Work out the finished part from the listing and answer in its coordinate system (mm). A direction names the side the tool comes from. Round coordinates to 2 decimals unless told otherwise and drop trailing zeros. Order: outer loops, then holes, each group sorted by start corner. A loop starts at its lowest first (then second) coordinate and runs counter-clockwise, first axis right, second up. Notation, with made-up numbers: M -6.5,-13.5 L 37.5,-13.5 A26 ccw 37.5,6.5 Z; hole C -16,-37 d3. An arc over 180 degrees is marked long. Return JSON: item names as keys, results as strings.
from build123d import *

# Parameters (mm, degrees)
SKETCH1_R           = 3.175
BOSS_EXTRUDE1_DEPTH = 88.9
CUT_EXTRUDE1_DEPTH  = 50.8
CUT_EXTRUDE2_START  = -6.5532
SKETCH3_R           = 3.175
SKETCH3_R_2         = 2.667
CUT_EXTRUDE2_DEPTH  = 0.7366


with BuildPart() as part:
    # Sketch1 → Boss-Extrude1 (new body)
    with BuildSketch(Plane(origin=(0, 0, 0), x_dir=(1, 0, 0), z_dir=(0, 1, 0))):
        Circle(SKETCH1_R)
    extrude(amount=BOSS_EXTRUDE1_DEPTH)

    # Sketch2 → Cut-Extrude1 (cut)
    with BuildSketch(Plane.XZ):
        Polygon((-2.5, 0), (-2.5, -1.957198253), (-3.175, -1.957198253), (-3.175, 1.957198253), (-2.5, 1.957198253), align=None)
    extrude(amount=-CUT_EXTRUDE1_DEPTH, mode=Mode.SUBTRACT)

    # Sketch3 → Cut-Extrude2 (cut)
    with BuildSketch(Plane(origin=(0, 88.9, 0), x_dir=(1, 0, 0), z_dir=(0, 1, 0)).offset(CUT_EXTRUDE2_START)):
        Circle(SKETCH3_R)
        Circle(SKETCH3_R_2, mode=Mode.SUBTRACT)
    extrude(amount=-CUT_EXTRUDE2_DEPTH, mode=Mode.SUBTRACT)


solid = part.part
Item 1: Which of the six approach directions +Z, -Z, +X, -X, +Y, -Y give full straight-line access (tool end or side, diameter ignored) to faces 1 (the flat face through (0, 88.9, 0)), 2 (the cylindrical face through (1.231, 81.984, 2.366))?
Output:
{"face 1": "+Z, -Z, +X, -X, +Y", "face 2": "none"}
Item 2: Find section A-A (z = 0). Determine the outline of the cut face in (x, y) (3 decimals), plus the area to 3 significant figures.
Output:
{"outline": "M -3.175,50.8 L -2.5,50.8 L -2.5,0 L 3.175,0 L 3.175,81.61 L 2.667,81.61 L 2.667,82.347 L 3.175,82.347 L 3.175,88.9 L -3.175,88.9 L -3.175,82.347 L -2.667,82.347 L -2.667,81.61 L -3.175,81.61 Z", "area": "529 mm^2"}
Item 3: Consider line 1 along X through (y, z) = (45.5, 1.75); line 2 along Y through (x, z) = (2.25, 2); line 3 along X through (y, z) = (33.5, -2.5). Determine where each line is inside the solid, lowest interval first. Write a range as [from, to].
Output:
{"line 1": "x = [-2.5, 2.65]", "line 2": "y = [0, 81.61], [82.35, 88.9]", "line 3": "x = [-1.96, 1.96]"}
Item 4: This flat-tipped pin is pushed along its axis until it touches: pin 1 (1.5 mm diameter, centred on x = 2.5, y = 72, fed in from +Z). Where does it stop, or does it pass through?
Output:
{"pin 1": "stops at z = 2.65"}
Item 5: Find section B-B (x = 1.75). Determine the outline of the cut face in (y, z).
Output:
{"outline": "M 0,-2.65 L 81.61,-2.65 L 81.61,-2.01 L 82.35,-2.01 L 82.35,-2.65 L 88.9,-2.65 L 88.9,2.65 L 82.35,2.65 L 82.35,2.01 L 81.61,2.01 L 81.61,2.65 L 0,2.65 Z"}
Item 6: The mould has two halves that part along Y. Classify faces 3 (the flat face through (-2.5, 25, 0)), 4 (the flat face through (0, 0, 0)), 5 (the flat face through (-2, 82.347, -2)): pulls with the +Y half, pulls with the -Y half, needs draft (parallel to the pull), parting line crosses it, or undercut.
Output:
{"face 3": "needs draft", "face 4": "pulls with the -Y half", "face 5": "undercut"}
Item 7: Find section C-C (y = 56). Determine the outline of the cut face in (x, z) (3 decimals).
Output:
{"outline": "C 0,0 d6.35"}
